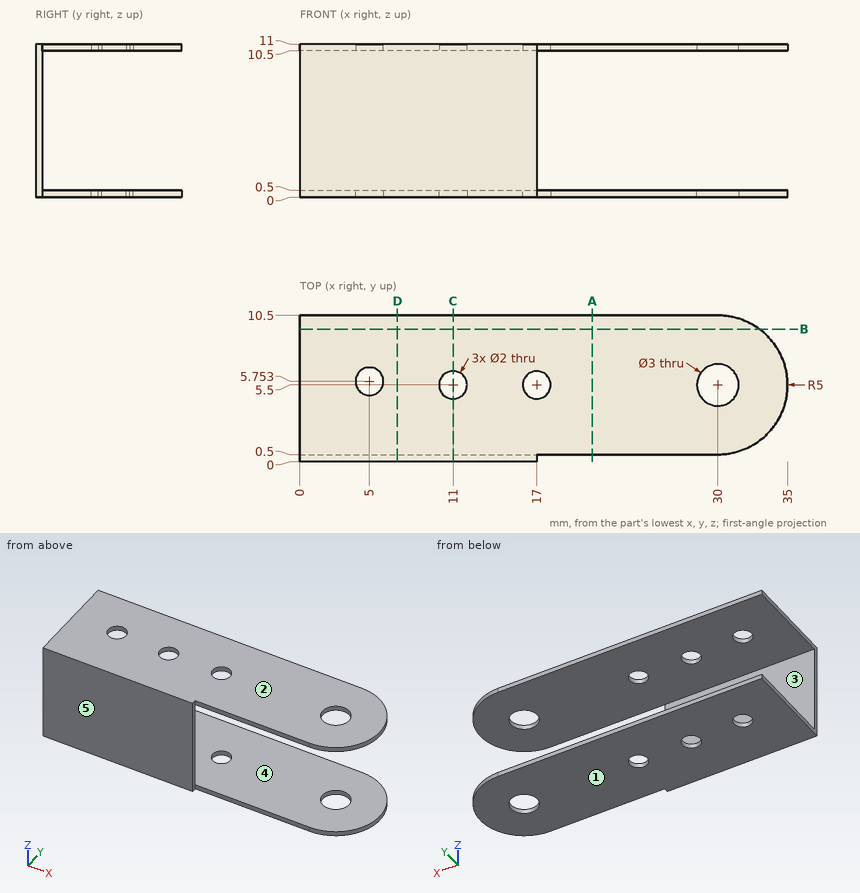
Source: three-view drawing plus pictorial views. Frame: mm from the lowest corner of the part. A direction names the side the tool comes from. Round coordinates to 2 decimals unless told otherwise and drop trailing zeros. Order: outer loops, then holes, each group sorted by start corner. A loop starts at its lowest first (then second) coordinate and runs counter-clockwise, first axis right, second up. Notation, with made-up numbers: (-21.5, 28) -> (-11.5, 28) arc R23 ccw to (-11.5, 66) -> close; hole circle Ø7 at (-3, 7). An arc over 180 degrees is marked (long way). Use one line per item in the form item = value.
(1) Section C-C on x = 11. Return loops of the section in (y, z), and give its area (3 significant figures).
Results list:
outline = (0, 0) -> (4.5, 0) -> (4.5, 0.5) -> (0.5, 0.5) -> (0.5, 10.5) -> (4.5, 10.5) -> (4.5, 11) -> (0, 11) -> close; (6.5, 0) -> (10.5, 0) -> (10.5, 0.5) -> (6.5, 0.5) -> close; (6.5, 10.5) -> (10.5, 10.5) -> (10.5, 11) -> (6.5, 11) -> close
area = 13.5 mm^2
(2) Section A-A on x = 21. Return loops of the section in (y, z), and give its area (3 significant figures).
Results list:
outline = (0.5, 0) -> (10.5, 0) -> (10.5, 0.5) -> (0.5, 0.5) -> close; (0.5, 10.5) -> (10.5, 10.5) -> (10.5, 11) -> (0.5, 11) -> close
area = 10.0 mm^2
(3) Section D-D on x = 7. Return loops of the section in (y, z).
Results list:
outline = (0, 0) -> (10.5, 0) -> (10.5, 0.5) -> (0.5, 0.5) -> (0.5, 10.5) -> (10.5, 10.5) -> (10.5, 11) -> (0, 11) -> close
(4) Ray query, probe 1 along Y at (x, z) = (11, 0.15); probe 2 along Z at (x, y) = (29.5, 10); probe 3 along Y at (x, z) = (5, 0.4). Return the intervals inside material, ascending. Write a range as [from, to].
Results list:
probe_1 = [0, 4.5], [6.5, 10.5]
probe_2 = [0, 0.5], [10.5, 11]
probe_3 = [0, 4.75], [6.75, 10.5]
(5) First-contact query: pin 1 Ø1.8 at (x, y) = (11, 5.5) entering from -Z; pin 2 Ø5 at (x, z) = (5.5, 3.5) entering from +Y; pin 3 Ø0.6 at (x, z) = (26.5, 0) entering from -Y. Flat tips, straight axial feed; report the tip coordinate or a pass-through.
Results list:
pin_1 = through
pin_2 = 0.5
pin_3 = 0.5
(6) Access query for the marked faces 4 and 5. Directions: +Z, -Z, +X, -X, +Y, -Y. A direction counts if a zero-diameter tool reaches every point of the face in a straight line with its end or side. Return the directions, or none.
Results list:
face_4 = +X, -X, +Y
face_5 = +Z, -Z, +X, -X, -Y
(7) Draft query along Z for the marked faces 1, 2 and 3. Return one class per face: pulls with the +Z half, pulls with the -Z half, needs draft (parallel to the pull), parting line crosses it, or undercut.
Results list:
face_1 = pulls with the -Z half
face_2 = pulls with the +Z half
face_3 = undercut
(8) Section B-B on y = 9.5. Return loops of the section in (x, z).
Results list:
outline = (0, 0) -> (33, 0) -> (33, 0.5) -> (0, 0.5) -> close; (0, 10.5) -> (33, 10.5) -> (33, 11) -> (0, 11) -> close
